The listing builds one solid part. Answer for the finished solid, in the listing's coordinates (mm). A direction names the side the tool comes from. Give positions to 0.01 mm unless a question says otherwise; leave off trailing zeros. Loops run counter-clockwise (first coordinate to the right, second up) from the corner with the lowest first, then second, coordinate; pieces in that order, holes last. Notation, with made-up numbers: (86, 9.5) - (105, 9.5) arc R26 ccw to (105, 26.5) - close; hole circle Ø10 at (27, 70.25). An arc over 180 degrees is marked (long way). One line per item, written item: value. Start each with the question number.
from build123d import *

# Parameters (mm, degrees)
F1_DEPTH    = 2
F2_W        = 1.3
F2_H        = 1.1
F2_W_2      = 2.5
F3_DEPTH    = 20
F4_T1_DEPTH = 1.3
F5_T4_DEPTH = 6.9651427749


# Not quite as in the source:
# - a fillet or chamfer that OpenCascade refuses, or shapes differently, is made with other operations: its cross-section is extruded or revolved along the edge and cut away or added


with BuildPart() as f1:
    # F0 (on Top) → F1 (new body)
    with BuildSketch(Plane.XY):
        with BuildLine():
            ThreePointArc((0, 3), (0.8786796564, 0.8786796564), (3, 0))
            Line((3, 0), (9, 0))
            ThreePointArc((9, 0), (11.1213203436, 0.8786796564), (12, 3))
            Line((12, 3), (12, 6))
            ThreePointArc((12, 6), (13.4644660941, 9.5355339059), (17, 11))
            Line((17, 11), (28.25, 11))
            Line((28.25, 11), (28.25, 11.65))
            Line((28.25, 11.65), (46, 11.65))
            Line((46, 11.65), (46, 17.65))
            Line((46, 17.65), (28.25, 17.65))
            Line((28.25, 17.65), (28.25, 21))
            Line((28.25, 21), (17, 21))
            ThreePointArc((17, 21), (13.4644660941, 22.4644660941), (12, 26))
            Line((12, 26), (12, 29))
            ThreePointArc((12, 29), (11.1213203436, 31.1213203436), (9, 32))
            Line((9, 32), (3, 32))
            ThreePointArc((3, 32), (0.8786796564, 31.1213203436), (0, 29))
            Line((0, 29), (0, 3))
        make_face()
        with BuildLine():
            ThreePointArc((3, 27.75), (1.75, 29), (3, 30.25))
            Line((3, 30.25), (9, 30.25))
            ThreePointArc((9, 30.25), (10.25, 29), (9, 27.75))
            Line((9, 27.75), (3, 27.75))
        make_face(mode=Mode.SUBTRACT)
    extrude(amount=F1_DEPTH)

    # F2 (on face) → F3 (cut)
    with BuildSketch(Plane.YZ.offset(46)):
        with Locations((13.1, 1.45)):
            Rectangle(F2_W, F2_H)
        with Locations((16.4, 0.55)):
            Rectangle(F2_W_2, F2_H)
    extrude(amount=-F3_DEPTH, mode=Mode.SUBTRACT)

    # F4: fillet of radius 2 on 1 edges, made by hand

    # F4_s2 → F4_t1 (join)
    with BuildSketch(Plane.XZ.offset(-13.75)):
        with BuildLine():
            ThreePointArc((26, 2), (26.7372482618, 1.1970613634), (27.7860571099, 0.9))
            Line((27.7860571099, 0.9), (26, 0.9))
            Line((26, 0.9), (26, 2))
        make_face()
    extrude(amount=F4_T1_DEPTH)

    # F5: fillet of radius 2 on 1 edges, made by hand


with BuildPart() as f5_tool2:
    # F5_s3 → F5_t4 (new body)
    with BuildSketch(Plane.XZ.offset(-17.65)):
        with BuildLine():
            ThreePointArc((26, 0), (26.7372482618, 0.8029386366), (27.7860571099, 1.1))
            Line((27.7860571099, 1.1), (26, 1.1))
            Line((26, 1.1), (26, 0))
        make_face()
    extrude(amount=F5_T4_DEPTH)

    split(bisect_by=Plane.XZ.offset(-13.75), keep=Keep.BOTTOM)


with BuildPart() as f1_1:
    add(f1.part)

    # F5_t1: union F5_tool2
    add(f5_tool2.part)


solid = f1_1.part
1. A cutting plane is placed at C-C (y = 16.5). Determine the outline of the cut face in (x, z), plus the area to 3 significant figures.
2. A cutting plane is placed at D-D (y = 10). Determine the outline of the cut face in (x, z), plus the area to 3 significant figures.
3. Flat-ended cylindrical pins translate along their axes: pin 1 (0.9 mm diameter, centred on x = 31, z = 0.5, fed in from +Y); pin 2 (1.2 mm diameter, centred on x = 37.5, y = 17, fed in from -Z); pin 3 (0.6 mm diameter, centred on x = 20, z = 1, fed in from -Y). Find the tip coordinate at first contact, or state that the pin passes through.
4. For faces 1 (the cylindrical face through (26.72, 13.11, 1.21)), 2 (the flat face through (6, 30.25, 1)), 3 (the flat face through (27.4, 17.65, 0.4)), determine the directions among +Z, -Z, +X, -X, +Y, -Y from which every point of the face is accessible in a straight line to the end or side of a thin tool.
5. A cutting plane is placed at B-B (x = 32). Determine the outline of the cut face in (y, z).
6. Find the intervals of material crossed by L1, parallel to Y at x = 39, z = 1.6; L2, parallel to Y at x = 20.5, z = 1.75; L3, parallel to X at y = 26, z = 0.3, in increasing order. Write a range as [from, to].
7. Determine the mould class of faces 4 (the cylindrical face through (10.25, 29.03, 0.99)), 5 (the flat face through (28.25, 19, 1)), 6 (the flat face through (12, 16, 0)), 7 (the cylindrical face through (1.75, 28.97, 0.99)) for opening direction X: released by +X, released by -X, zero draft, split by the parting line, or undercut.
8. A cutting plane is placed at A-A (z = 1.6). Determine the outline of the cut face in (x, y), plus the area to 3 significant figures.
Results below:
1. outline: (0, 0) - (26, 0) arc R2 cw to (27.79, 1.1) - (46, 1.1) - (46, 2) - (0, 2) - close
1. area: 70.6 mm^2
2. outline: (0, 0) - (14, 0) - (14, 2) - (0, 2) - close
2. area: 28.0 mm^2
3. pin 1: stops at y = 15.15
3. pin 2: stops at z = 1.1
3. pin 3: stops at y = 11
4. face 1: +Z, +X
4. face 2: +Z, -Z
4. face 3: -Z, +X
5. outline: (11.65, 0) - (15.15, 0) - (15.15, 1.1) - (17.65, 1.1) - (17.65, 2) - (13.75, 2) - (13.75, 0.9) - (12.45, 0.9) - (12.45, 2) - (11.65, 2) - close
6. L1: y = [11.65, 12.45], [13.75, 17.65]
6. L2: y = [11, 21]
6. L3: x = [0, 12]
7. face 4: undercut
7. face 5: released by +X
7. face 6: zero draft
7. face 7: undercut
8. outline: (0, 3) arc R3 ccw to (3, 0) - (9, 0) arc R3 ccw to (12, 3) - (12, 6) arc R5 cw to (17, 11) - (28.25, 11) - (28.25, 11.65) - (46, 11.65) - (46, 12.45) - (26.27, 12.45) - (26.27, 13.75) - (46, 13.75) - (46, 17.65) - (28.25, 17.65) - (28.25, 21) - (17, 21) arc R5 cw to (12, 26) - (12, 29) arc R3 ccw to (9, 32) - (3, 32) arc R3 ccw to (0, 29) - close; hole (3, 27.75) - (9, 27.75) arc R1.25 ccw to (9, 30.25) - (3, 30.25) arc R1.25 ccw to start
8. area: 610 mm^2
